Verification items for the finished model (mm, model axes). A direction names the side the tool comes from. Round coordinates to 2 decimals unless told otherwise and drop trailing zeros. Write each loop counter-clockwise with the first axis right and the second up, starting at its lowest first coordinate (ties: lowest second). Pieces come first, ordered by that corner, then holes. Notation, with made-up numbers: M 16.25,52 L 61.25,52 A8 ccw 61.25,59 Z; hole C 24.5,-6.75 d3. An arc over 180 degrees is marked long. Answer in a Markdown table with one row per item. Add a question column.
1. Set-up check for faces 1 (the flat face through (399, -33, -20)), 2 (the flat face through (625, 0, -20)), 3 (the flat face through (795, 0, 26)), 4 (the flat face through (406, -8, -18)), 5 (the flat face through (180, 0, -20)): record each of +Z, -Z, +X, -X, +Y, -Y from which the full face is reachable in a straight line by a thin tool's end or side.
2. Material ranges on probe 1 along Z at (x, y) = (50, -19.4); probe 2 along Y at (x, z) = (714, -3); probe 3 along Y at (x, z) = (432.5, -21.25), recorded low to high.
3. Go/stop test with flat-tipped pins: pin 1 Ø10.5 at (x, y) = (600, 0) entering from +Z; pin 2 Ø7.5 at (x, y) = (415, -32) entering from +Z; pin 3 Ø11 at (x, z) = (580, 8.5) entering from -Y. Record where each tip stops, or that it passes through.
4. Sectioned sample at A-A on x = 515. Record the cut outline in (y, z), plus the area to 3 significant figures.
5. Draft check along Z on faces 6 (the flat face through (406, 18, 0)), 7 (the cylindrical face through (393.323, -2.103, -21.451)), 8 (the flat face through (406, 0, 18)), 9 (the flat face through (399, 32, -20)). Enter one of: pulls with the +Z half, pulls with the -Z half, needs draft (parallel to the pull), parting line crosses it, or undercut.
```python
from build123d import *

# Parameters (mm, degrees)
F0_W      = 40
F0_H      = 40
F0_W_2    = 36
F0_H_2    = 36
F1_DEPTH  = 400
F2_W      = 40
F2_H      = 60
F3_DEPTH  = 5
F4_D      = 6.4
F6_D      = 6.5
F8_D      = 3.2
F9_D      = 8
F10_D     = 6.5
F13_W     = 90
F13_H     = 25
F13_H_2   = 40
F14_DEPTH = 5
F16_D     = 6.5
F17_D     = 14
F17_DEPTH = 10
F17_TIP   = 4.2060243332


with BuildPart() as f1:
    # F0 (on Right) → F1 (new body)
    with BuildSketch(Plane.YZ):
        Rectangle(F0_W, F0_H)
        Rectangle(F0_W_2, F0_H_2, mode=Mode.SUBTRACT)
    extrude(amount=F1_DEPTH)

    # F2 (on Right) → F3 (join)
    with BuildSketch(Plane.YZ):
        with Locations((0, 10)):
            Rectangle(F2_W, F2_H)
    extrude(amount=F3_DEPTH)

    # F4 (through all)
    with Locations(Plane(origin=(0, 0, 0), x_dir=(0, 1, 0), z_dir=(-1, 0, 0))):
        with Locations((0, -30)):
            Hole(F4_D / 2)

    # F6 (through all)
    with Locations(Plane.XY.offset(20)):
        with Locations((165, 0), (200, 0)):
            Hole(F6_D / 2)

    # F8 (through all)
    with Locations(Plane.XZ.offset(20)):
        with Locations((50, 10), (50, -10), (300, 10), (300, -10)):
            Hole(F8_D / 2)

    # F9 (through all)
    with Locations(Plane(origin=(0, 0, 0), x_dir=(0, 1, 0), z_dir=(-1, 0, 0))):
        with Locations((0, 0)):
            Hole(F9_D / 2)

    # F10 (through all)
    with Locations(Plane.XZ.offset(20)):
        with Locations((100, 0)):
            Hole(F10_D / 2)

    # F12: F1 across face


with BuildPart() as f1_1:
    add(f1.part)
    add(f1.part.mirror(Plane.YZ.offset(400)))

    # F13 (on face) → F14 (join)
    with BuildSketch(Plane(origin=(0, 0, -20), x_dir=(1, 0, 0), z_dir=(0, 0, -1))):
        with Locations((400, 32.5)):
            Rectangle(F13_W, F13_H)
        with Locations((400, -32.5)):
            Rectangle(F13_W, F13_H)
        with Locations((400, 0)):
            Rectangle(F13_W, F13_H_2)
    extrude(amount=F14_DEPTH)

    # F16 (through all)
    with Locations(Plane(origin=(0, 0, -25), x_dir=(1, 0, 0), z_dir=(0, 0, -1))):
        with Locations((367.5, 32.5), (432.5, 32.5), (432.5, -32.5), (367.5, -32.5)):
            Hole(F16_D / 2)

    # F17
    with Locations(Plane(origin=(0, 0, -25), x_dir=(1, 0, 0), z_dir=(0, 0, -1))):
        with Locations((400, 0)):
            Hole(F17_D / 2, depth=F17_DEPTH)
            with Locations((0, 0, -(F17_DEPTH + F17_TIP / 2))):  # 118° drill point
                Cone(0, F17_D / 2, F17_TIP, mode=Mode.SUBTRACT)


solid = f1_1.part
```
Geometry check:
| question | item | result |
|---|---|---|
| 1 | face 1 | +Z, +X, -X, -Y |
| 1 | face 2 | -Z, +X, +Y, -Y |
| 1 | face 3 | +Z, +Y, -Y |
| 1 | face 4 | none |
| 1 | face 5 | -Z, -X, +Y, -Y |
| 2 | probe 1 | z = -20 to -11.6, -8.4 to 8.4, 11.6 to 20 |
| 2 | probe 2 | y = -20 to -18, 18 to 20 |
| 2 | probe 3 | y = -45 to -35.75, -29.25 to 29.25, 35.75 to 45 |
| 3 | pin 1 | stops at z = 20 |
| 3 | pin 2 | stops at z = -20 |
| 3 | pin 3 | stops at y = -20 |
| 4 | outline | M -20,-20 L 20,-20 L 20,20 L -20,20 Z; hole M -18,-18 L 18,-18 L 18,18 L -18,18 Z |
| 4 | area | 304 mm2 |
| 5 | face 6 | undercut |
| 5 | face 7 | needs draft |
| 5 | face 8 | undercut |
| 5 | face 9 | pulls with the +Z half |
